from build123d import *

# Parameters (mm, degrees)
SALIENTE_EXTRUIR1_DEPTH = 10
CROQUIS2_R              = 2
CORTAR_EXTRUIR1_DEPTH   = 18
MATRIZC1_COUNT          = 6
CROQUIS4_R              = 11.25
SALIENTE_EXTRUIR2_DEPTH = 36
CROQUIS5_R              = 6
CORTAR_EXTRUIR2_DEPTH   = 53


with BuildPart() as part:
    # Croquis1 → Saliente-Extruir1 (new body)
    with BuildSketch(Plane.XY):
        with BuildLine():
            Line((-8.714212529, -15.75), (8.714212529, -15.75))
            ThreePointArc((8.714212529, -15.75), (18, 0), (8.714212529, 15.75))
            Line((8.714212529, 15.75), (-8.714212529, 15.75))
            ThreePointArc((-8.714212529, 15.75), (-18, 0), (-8.714212529, -15.75))
        make_face()
    extrude(amount=SALIENTE_EXTRUIR1_DEPTH)

    # Croquis2 → Cortar-Extruir1 (cut)
    with BuildSketch(Plane.XY.offset(10)):
        with Locations((-15, 0)):
            Circle(CROQUIS2_R)
    cortar_extruir1 = extrude(amount=-CORTAR_EXTRUIR1_DEPTH, mode=Mode.SUBTRACT)

    # MatrizC1: Cortar-Extruir1 ×6 about axis
    matrizc1_axis = Axis((0.197930151, 0, 0), (0, 0, 1))
    for i in range(1, MATRIZC1_COUNT):
        add(cortar_extruir1.rotate(matrizc1_axis, i * 360 / MATRIZC1_COUNT), mode=Mode.SUBTRACT)

    # Croquis4 → Saliente-Extruir2 (add)
    with BuildSketch(Plane(origin=(0, 0, 0), x_dir=(-1, 0, 0), z_dir=(0, 0, -1))):
        with Locations(Location((0, 0, 0), (0, 0, 180))):
            Circle(CROQUIS4_R)
    extrude(amount=SALIENTE_EXTRUIR2_DEPTH)

    # Croquis5 → Cortar-Extruir2 (cut)
    with BuildSketch(Plane.XY.offset(10)):
        Circle(CROQUIS5_R)
    extrude(amount=-CORTAR_EXTRUIR2_DEPTH, mode=Mode.SUBTRACT)


solid = part.part
Build history of the part. All positions in model axes, mm. A direction names the side the tool comes from. Coordinates: 2 decimals unless noted, no trailing zeros. Write each loop counter-clockwise with the first axis right and the second up, starting at its lowest first coordinate (ties: lowest second). Pieces come first, ordered by that corner, then holes. Notation, with made-up numbers: (42, 47) -> (92, 47) arc R30 ccw to (92, 72) -> close; hole circle Ø1 at (-22.75, 23.5). An arc over 180 degrees is marked (long way). Use CSV: the item, a comma, the result in double quotes. Start each with the question number.
Q1. Pull direction Y, two halves, no side cores. Call faces 1 (the flat face through (0, 7, 10)), 2 (the cylindrical face through (13.49, -0.6, 5.07)), 3 (the cylindrical face through (-5.814, 14.379, 5.07)), 4 (the flat face through (0, 15.75, 5)): released by +Y, released by -Y, zero draft, split by the parting line, or undercut.
Q2. Cut at D-D, the plane z = -10. List the corners of the cut face in (x, y).
Q3. Cut at C-C, the plane y = -12.5. List the corners of the cut face in (x, z), then the cut area to 3 significant figures.
Q4. Cut at A-A, the plane x = 0. List the corners of the cut face in (y, z).
Q5. Cut at B-B, the plane y = 0. List the corners of the cut face in (x, z), then the cut area to 3 significant figures.
Q6. Drill centre lines: probe 1 along Y at (x, z) = (8, 3); probe 2 along Y at (x, z) = (8.5, 4); probe 3 along Z at (x, y) = (-10.5, 5.5). Where is each one in solid material? Low to high.
Q7. Flat gauge pins, fed straight in: pin 1 Ø3 at (x, y) = (7.8, 13.16) entering from -Z; pin 2 Ø5 at (x, y) = (-12, 10.5) entering from -Z; pin 3 Ø6 at (x, z) = (-7, -20) entering from -Y; pin 4 Ø5 at (x, y) = (15.4, 0) entering from +Z. Where does each tip first touch, or does it go through?
Q8. 3-axis set-ups, long thin cutter, end or side, ignore diameter. For faces 5 (the flat face through (-4, 11, 0)), 6 (the cylindrical face through (-18, 0, 5)): which of +Z, -Z, +X, -X, +Y, -Y reach the whole face in a straight line?
Checked values:
1,face 1,"zero draft"
1,face 2,"undercut"
1,face 3,"undercut"
1,face 4,"released by +Y"
2,outline,"circle Ø22.5 at (0, 0); hole circle Ø12 at (0, 0)"
3,outline,"(-12.95, 0) -> (-9.29, 0) -> (-9.29, 10) -> (-12.95, 10) -> close; (-5.51, 0) -> (5.91, 0) -> (5.91, 10) -> (-5.51, 10) -> close; (9.68, 0) -> (12.95, 0) -> (12.95, 10) -> (9.68, 10) -> close"
3,area,"184 mm²"
4,outline,"(-15.75, 0) -> (-11.25, 0) -> (-11.25, -36) -> (-6, -36) -> (-6, 10) -> (-15.75, 10) -> close; (6, -36) -> (11.25, -36) -> (11.25, 0) -> (15.75, 0) -> (15.75, 10) -> (6, 10) -> close"
5,outline,"(-18, 0) -> (-17, 0) -> (-17, 10) -> (-18, 10) -> close; (-13, 0) -> (-11.25, 0) -> (-11.25, -36) -> (-6, -36) -> (-6, 10) -> (-13, 10) -> close; (6, -36) -> (11.25, -36) -> (11.25, 0) -> (13.4, 0) -> (13.4, 10) -> (6, 10) -> close; (17.4, 0) -> (18, 0) -> (18, 10) -> (17.4, 10) -> close"
5,area,"538 mm²"
6,probe 1,"y = -15.75 to -15.15, -11.17 to 11.17, 15.15 to 15.75"
6,probe 2,"y = -15.75 to -15.03, -11.29 to 11.29, 15.03 to 15.75"
6,probe 3,"z = 0 to 10"
7,pin 1,"passes through"
7,pin 2,"stops at z = 0"
7,pin 3,"stops at y = -10.51"
7,pin 4,"stops at z = 10"
8,face 5,"-Z"
8,face 6,"+Z, -Z, -X"
